Geometry: final body of the model. Coordinates: model frame, mm. A direction names the side the tool comes from. Give positions to 0.01 mm unless a question says otherwise; leave off trailing zeros. Loops run counter-clockwise (first coordinate to the right, second up) from the corner with the lowest first, then second, coordinate; pieces in that order, holes last.
1. Section B-B, the plane x = 5.5. Output: boundary loops of the cut face in (y, z).
2. Material intervals for line 1 along Z through (x, y) = (3.5, 5); line 2 along X through (y, z) = (5.75, -9.5); line 3 along X through (y, z) = (4, 14), sorted ascending.
3. Section C-C, the plane x = -0.5. Output: boundary loops of the cut face in (y, z), then the cut area to 3 significant figures.
4. First-contact query: P1, Ø6, axis at x = 0.5, z = 10, coming from the -Y side. Flat tip, straight axial feed; report the tip coordinate or a pass-through.
5. Section D-D, the plane y = 6.5. Output: boundary loops of the cut face in (x, z) (3 decimals), then the cut area to 3 significant figures.
6. Access query for faces 5 (the face through (0, 5, -16.9)), 6 (the face through (7, 5, 0)). Directions: +Z, -Z, +X, -X, +Y, -Y. A direction counts if a zero-diameter tool reaches every point of the face in a straight line with its end or side. Return the directions, or none.
7. Draft query along Z for faces 1 (the face through (0, 5, 12)), 2 (the face through (-7, 5, 0)), 3 (the face through (-7.2, 0, -1.2)), 4 (the face through (0, 5, 16.9)). Return one class per face: +Z half, -Z half, draft (parallel to the pull), parting line (faces both ways), or undercut.
8. Section A-A, the plane z = -11. Output: boundary loops of the cut face in (x, y), then the cut area to 3 significant figures.
Autodesk Inventor part; units mm, degrees
ref_plane "YZ Plane" through (0, 0, 0) normal (1, 0, 0) x (0, 1, 0)
ref_plane "XZ Plane" through (0, 0, 0) normal (0, 1, 0) x (-1, 0, 0)
ref_plane "XY Plane" through (0, 0, 0) normal (0, 0, 1) x (1, 0, 0)
sketch "Sketch2" plane through (0, 0, 0) normal (0, 1, 0) x (-1, 0, 0)
  line L0 (8.14, 16.9) -> (-8.14, 16.9)
  line L1 (-8.14, 16.9) -> (-8.14, -16.9)
  line L2 (-8.14, -16.9) -> (8.14, -16.9)
  line L3 (8.14, -16.9) -> (8.14, 16.9)
  line L4 (8.14, 16.9) -> (-8.14, -16.9) construction
  line L5 (-8.14, 16.9) -> (8.14, -16.9) construction
  point P0 (0, 0)
  dimension "d0" = 33.8
  dimension "d1" = 16.28
sketch "Sketch3" plane through (0, 0, 0) normal (0, 1, 0) x (-1, 0, 0)
  line L0 (-7, -12) -> (7, -12)
  line L1 (7, -12) -> (7, 12)
  line L2 (7, 12) -> (-7, 12)
  line L3 (-7, 12) -> (-7, -12)
  line L4 (-7, -12) -> (7, 12) construction
  line L5 (7, -12) -> (-7, 12) construction
  point P0 (0, 0)
  dimension "d2" = 24
  dimension "d3" = 14
extrude "Extrusion1" add sketch "Sketch2" along normal blind 10
extrude "Extrusion2" cut sketch "Sketch3" along normal blind 10
sketch "Sketch5" plane through (0, 10, 0) normal (0, 1, 0) x (1, 0, 0)
  line L0 (7, -12) -> (-7, -12)
  point P0 (0, 0)
  point P1 (0.476, -14)
  dimension "d22" = 2
hole "Hole1" at (0.476, 10, 14) direction (0, -1, 0) diameter 3.81 depth 10
sketch "Sketch6" plane through (0, 10, 0) normal (0, 1, 0) x (1, 0, 0)
  line L0 (7, 12) -> (-7, 12)
  point P0 (0, 0)
  point P1 (0.8061, 14)
  dimension "d30" = 2
hole "Hole2" at (0.8061, 10, -14) direction (0, -1, 0) diameter 3.81 depth 10
properties part number "servo housing electric boogaloo"
Answers below:
1. outline: (0, -16.9) - (10, -16.9) - (10, -12) - (0, -12) - close; (0, 12) - (10, 12) - (10, 16.9) - (0, 16.9) - close
2. line 1: z = -16.9 to -12, 12 to 16.9
2. line 2: x = -8.14 to -7, 7 to 8.14
2. line 3: x = -8.14 to -1.43, 2.38 to 8.14
3. outline: (0, -16.9) - (10, -16.9) - (10, -15.39) - (0, -15.39) - close; (0, -12.61) - (10, -12.61) - (10, -12) - (0, -12) - close; (0, 12) - (10, 12) - (10, 12.36) - (0, 12.36) - close; (0, 15.64) - (10, 15.64) - (10, 16.9) - (0, 16.9) - close
3. area: 37.5 mm2
4. P1: stops at y = 0
5. outline: (-8.14, -16.9) - (8.14, -16.9) - (8.14, 16.9) - (-8.14, 16.9) - close; hole (-7, -12) - (7, -12) - (7, 12) - (-7, 12) - close; hole circle Ø3.81 at (0.476, 14); hole circle Ø3.81 at (0.806, -14)
5. area: 191 mm2
6. face 5: -Z, +X, -X, +Y, -Y
6. face 6: +Y, -Y
7. face 1: undercut
7. face 2: undercut
7. face 3: draft
7. face 4: +Z half
8. outline: (-8.14, 0) - (-7, 0) - (-7, 10) - (-8.14, 10) - close; (7, 0) - (8.14, 0) - (8.14, 10) - (7, 10) - close
8. area: 22.8 mm2
